from build123d import *

# Parameters (mm, degrees)
SKETCH1_W           = 13.101477715
SKETCH1_H           = 14.558194743
SKETCH1_W_2         = 8.5
SKETCH1_H_2         = 10.5
SKETCH1_W_3         = 16.678859494
SKETCH1_H_3         = 17.418317903
SKETCH1_W_4         = 15.995214615
SKETCH1_H_4         = 12.7738
SKETCH1_W_5         = 12.8
SKETCH1_H_5         = 13.82
BOSS_EXTRUDE1_DEPTH = 1


with BuildPart() as part:
    # Sketch1 → Boss-Extrude1 (new body)
    with BuildSketch(Plane.XY):
        with BuildLine():
            Line((-51.940144553, -23.805569529), (62.059855447, -23.805569529))
            ThreePointArc((62.059855447, -23.805569529), (64.18117579, -22.926889873), (65.059855447, -20.805569529))
            Line((65.059855447, -20.805569529), (65.059855447, 0.194430471))
            Line((65.059855447, 0.194430471), (65.059855447, 21.194430471))
            ThreePointArc((65.059855447, 21.194430471), (64.18117579, 23.315750814), (62.059855447, 24.194430471))
            Line((62.059855447, 24.194430471), (-51.940144553, 24.194430471))
            ThreePointArc((-51.940144553, 24.194430471), (-54.061464897, 23.315750814), (-54.940144553, 21.194430471))
            Line((-54.940144553, 21.194430471), (-54.940144553, 0.194430471))
            Line((-54.940144553, 0.194430471), (-54.940144553, -20.805569529))
            ThreePointArc((-54.940144553, -20.805569529), (-54.061464897, -22.926889873), (-51.940144553, -23.805569529))
        make_face()
        with Locations((0.968394625, 2.55037109)):
            Rectangle(SKETCH1_W, SKETCH1_H, mode=Mode.SUBTRACT)
        with Locations((-35.690144553, 5.119430471)):
            Rectangle(SKETCH1_W_2, SKETCH1_H_2, mode=Mode.SUBTRACT)
        with Locations((-17.6295743, 1.82407152)):
            Rectangle(SKETCH1_W_3, SKETCH1_H_3, mode=Mode.SUBTRACT)
        with Locations((35.50746287, 3.606330471)):
            Rectangle(SKETCH1_W_4, SKETCH1_H_4, mode=Mode.SUBTRACT)
        with Locations((18.059855447, 2.659430471)):
            Rectangle(SKETCH1_W_5, SKETCH1_H_5, mode=Mode.SUBTRACT)
    extrude(amount=BOSS_EXTRUDE1_DEPTH)


solid = part.part
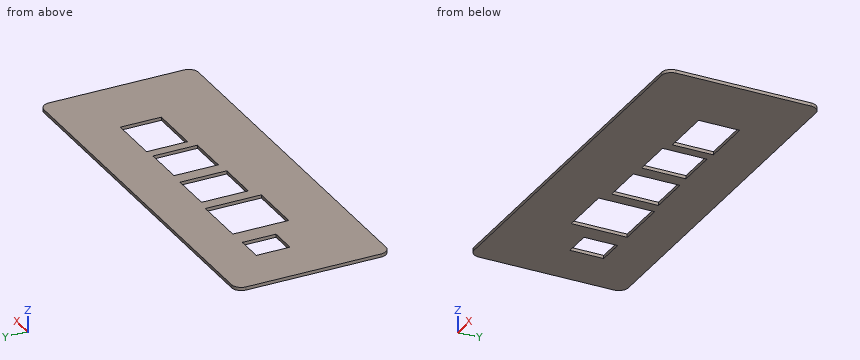
CAD build for the part. Positions are in the model's coordinates, mm. Round coordinates to 2 decimals unless told otherwise and drop trailing zeros. Order: outer loops, then holes, each group sorted by start corner. A loop starts at its lowest first (then second) coordinate and runs counter-clockwise, first axis right, second up. Notation, with made-up numbers: (0.5, 66) -> (30.5, 66) arc R21 cw to (30.5, 73) -> close; hole circle Ø5 at (3, 46.5). An arc over 180 degrees is marked (long way). Write item = value, one per line. Start each with the question number.
(1) Cut at C-C, the plane z = 0.6. List the corners of the cut face in (x, y).
(2) Probe line 1 (X direction, y = 0.5, z = 0.9); line 2 (X direction, y = -0.5, z = 0.25); line 3 (Y direction, x = 24, z = 0.4). List the from-to ranges inside material, lowest first. Write a range as [from, to].
(3) Cut at A-A, the plane y = 7. List the corners of the cut face in (x, z).
(4) Cut at B-B, the plane x = 29. List the corners of the cut face in (y, z), then the cut area to 3 significant figures.
(5) Cut at D-D, the plane x = -24. List the corners of the cut face in (y, z), then the cut area to 3 significant figures.
Model answer:
q1.outline = (-54.94, -20.81) arc R3 ccw to (-51.94, -23.81) -> (62.06, -23.81) arc R3 ccw to (65.06, -20.81) -> (65.06, 21.19) arc R3 ccw to (62.06, 24.19) -> (-51.94, 24.19) arc R3 ccw to (-54.94, 21.19) -> close; hole (-39.94, -0.13) -> (-31.44, -0.13) -> (-31.44, 10.37) -> (-39.94, 10.37) -> close; hole (-25.97, -6.89) -> (-9.29, -6.89) -> (-9.29, 10.53) -> (-25.97, 10.53) -> close; hole (-5.58, -4.73) -> (7.52, -4.73) -> (7.52, 9.83) -> (-5.58, 9.83) -> close; hole (11.66, -4.25) -> (24.46, -4.25) -> (24.46, 9.57) -> (11.66, 9.57) -> close; hole (27.51, -2.78) -> (43.51, -2.78) -> (43.51, 9.99) -> (27.51, 9.99) -> close
q2.line_1 = [-54.94, -39.94], [-31.44, -25.97], [-9.29, -5.58], [7.52, 11.66], [24.46, 27.51], [43.51, 65.06]
q2.line_2 = [-54.94, -25.97], [-9.29, -5.58], [7.52, 11.66], [24.46, 27.51], [43.51, 65.06]
q2.line_3 = [-23.81, -4.25], [9.57, 24.19]
q3.outline = (-54.94, 0) -> (-39.94, 0) -> (-39.94, 1) -> (-54.94, 1) -> close; (-31.44, 0) -> (-25.97, 0) -> (-25.97, 1) -> (-31.44, 1) -> close; (-9.29, 0) -> (-5.58, 0) -> (-5.58, 1) -> (-9.29, 1) -> close; (7.52, 0) -> (11.66, 0) -> (11.66, 1) -> (7.52, 1) -> close; (24.46, 0) -> (27.51, 0) -> (27.51, 1) -> (24.46, 1) -> close; (43.51, 0) -> (65.06, 0) -> (65.06, 1) -> (43.51, 1) -> close
q4.outline = (-23.81, 0) -> (-2.78, 0) -> (-2.78, 1) -> (-23.81, 1) -> close; (9.99, 0) -> (24.19, 0) -> (24.19, 1) -> (9.99, 1) -> close
q4.area = 35.2 mm2
q5.outline = (-23.81, 0) -> (-6.89, 0) -> (-6.89, 1) -> (-23.81, 1) -> close; (10.53, 0) -> (24.19, 0) -> (24.19, 1) -> (10.53, 1) -> close
q5.area = 30.6 mm2
